```python
from build123d import *

# Parameters (mm, degrees)
F0_W     = 77.3
F0_H     = 25.4
F1_DEPTH = 2
F3_D     = 5.5
F4_R     = 5


with BuildPart() as f1:
    # F0 (on Top) → F1 (new body)
    with BuildSketch(Plane.XY):
        with Locations((38.65, 12.7)):
            Rectangle(F0_W, F0_H)
    extrude(amount=F1_DEPTH)

    # F3 (through all)
    with Locations(Plane.XY.offset(2)):
        with Locations((10, 12.7), (40, 12.7), (60, 12.7)):
            Hole(F3_D / 2)

    # F4
    f4_edges = [f1.edges().sort_by_distance(p)[0] for p in [
        (0, 25.4, 1),
        (0, 0, 1),
        (77.3, 0, 1),
        (77.3, 25.4, 1),
    ]]
    fillet(f4_edges, radius=F4_R)


solid = f1.part
```
Check sheet for the modelled part. Datum: model origin and axes. Units: mm. Round coordinates to 2 decimals unless told otherwise and drop trailing zeros. Loops run counter-clockwise (first coordinate to the right, second up) from the corner with the lowest first, then second, coordinate; pieces in that order, holes last. Notation, with made-up numbers: (9, -3.5) -> (63, -3.5) arc R21 ccw to (63, 3.5) -> close; hole circle Ø6 at (-21, 18.5). An arc over 180 degrees is marked (long way). Write item = value, one per line. Start each with the question number.
1) Sectioned sample at C-C, the plane x = 60. Record the cut outline in (y, z), plus the area to 3 significant figures.
2) Gauge pin test, flat end, axial feed: pin 1 Ø7 at (x, y) = (60, 12.7) entering from +Z. Record the tip position at first contact, or that the pin passes through.
3) Sectioned sample at D-D, the plane x = 12. Record the cut outline in (y, z), plus the area to 3 significant figures.
4) Release check for a two-part mould opening along X. For faces 1 (the cylindrical face through (1, 2, 1)), 2 (the cylindrical face through (8.52, 15.02, 0.99)), 3 (the flat face through (77.3, 13, 1)) record: released by +X, released by -X, zero draft, split by the parting line, or undercut.
5) Sectioned sample at A-A, the plane z = 1.4. Record the cut outline in (x, y), plus the area to 3 significant figures.
6) Sectioned sample at B-B, the plane y = 12.7. Record the cut outline in (x, z), plus the area to 3 significant figures.
7) Thickness scan on probe 1 along Y at (x, z) = (10, 0.6); probe 2 along X at (y, z) = (14.75, 1.5); probe 3 along Y at (x, z) = (61.5, 1.25). Record the ranges inside material, lowest first.
Results are:
q1.outline = (0, 0) -> (9.95, 0) -> (9.95, 2) -> (0, 2) -> close; (15.45, 0) -> (25.4, 0) -> (25.4, 2) -> (15.45, 2) -> close
q1.area = 39.8 mm^2
q2.pin_1 = 2
q3.outline = (0, 0) -> (10.81, 0) -> (10.81, 2) -> (0, 2) -> close; (14.59, 0) -> (25.4, 0) -> (25.4, 2) -> (14.59, 2) -> close
q3.area = 43.3 mm^2
q4.face_1 = released by -X
q4.face_2 = undercut
q4.face_3 = released by +X
q5.outline = (0, 5) arc R5 ccw to (5, 0) -> (72.3, 0) arc R5 ccw to (77.3, 5) -> (77.3, 20.4) arc R5 ccw to (72.3, 25.4) -> (5, 25.4) arc R5 ccw to (0, 20.4) -> close; hole circle Ø5.5 at (10, 12.7); hole circle Ø5.5 at (40, 12.7); hole circle Ø5.5 at (60, 12.7)
q5.area = 1,870 mm^2
q6.outline = (0, 0) -> (7.25, 0) -> (7.25, 2) -> (0, 2) -> close; (12.75, 0) -> (37.25, 0) -> (37.25, 2) -> (12.75, 2) -> close; (42.75, 0) -> (57.25, 0) -> (57.25, 2) -> (42.75, 2) -> close; (62.75, 0) -> (77.3, 0) -> (77.3, 2) -> (62.75, 2) -> close
q6.area = 122 mm^2
q7.probe_1 = 0 to 9.95, 15.45 to 25.4
q7.probe_2 = 0 to 8.17, 11.83 to 38.17, 41.83 to 58.17, 61.83 to 77.3
q7.probe_3 = 0 to 10.4, 15 to 25.4
